Source: three-view drawing plus pictorial views. Frame: mm from the lowest corner of the part. A direction names the side the tool comes from. Give positions to 0.01 mm unless a question says otherwise; leave off trailing zeros. Order: outer loops, then holes, each group sorted by start corner. A loop starts at its lowest first (then second) coordinate and runs counter-clockwise, first axis right, second up. Notation, with made-up numbers: M 47.5,60.5 L 97.5,60.5 A19 ccw 97.5,84.5 Z; hole C -37,83 d9. An arc over 180 degrees is marked long. Use CSV: the item, a comma, the result in double quotes. Start each with the question number.
Item 1: First-contact query: pin 1 (4.5 mm diameter, centred on x = 11.575, y = 8.875, fed in from +Z); pin 2 (0.5 mm diameter, centred on x = 16, y = 9, fed in from +Z); pin 3 (2 mm diameter, centred on y = 17, z = 3, fed in from -X). Flat tips, straight axial feed; report the tip coordinate or a pass-through.
Item 2: Access query for the marked faces 1 and 2. Directions: +Z, -Z, +X, -X, +Y, -Y. A direction counts if a zero-diameter tool reaches every point of the face in a straight line with its end or side. Return the directions, or none.
Item 3: Ray query, probe 1 along X at (y, z) = (18.5, 2.9); probe 2 along Y at (x, z) = (13.25, 1.6); probe 3 along X at (y, z) = (9.25, 3.95). Return the intervals inside material, ascending. Write a range as from..to.
Item 4: Section query B-B on x = 12.5. Return loops of the section in (y, z).
Item 5: Section query C-C on y = 10.75. Return loops of the section in (x, z).
Item 6: Pull-direction query (X, two-part tool) for the marked faces 3, 4, 5 and 6; classes: +X half, -X half, draft (parallel to the pull), parting line (faces both ways), or undercut.
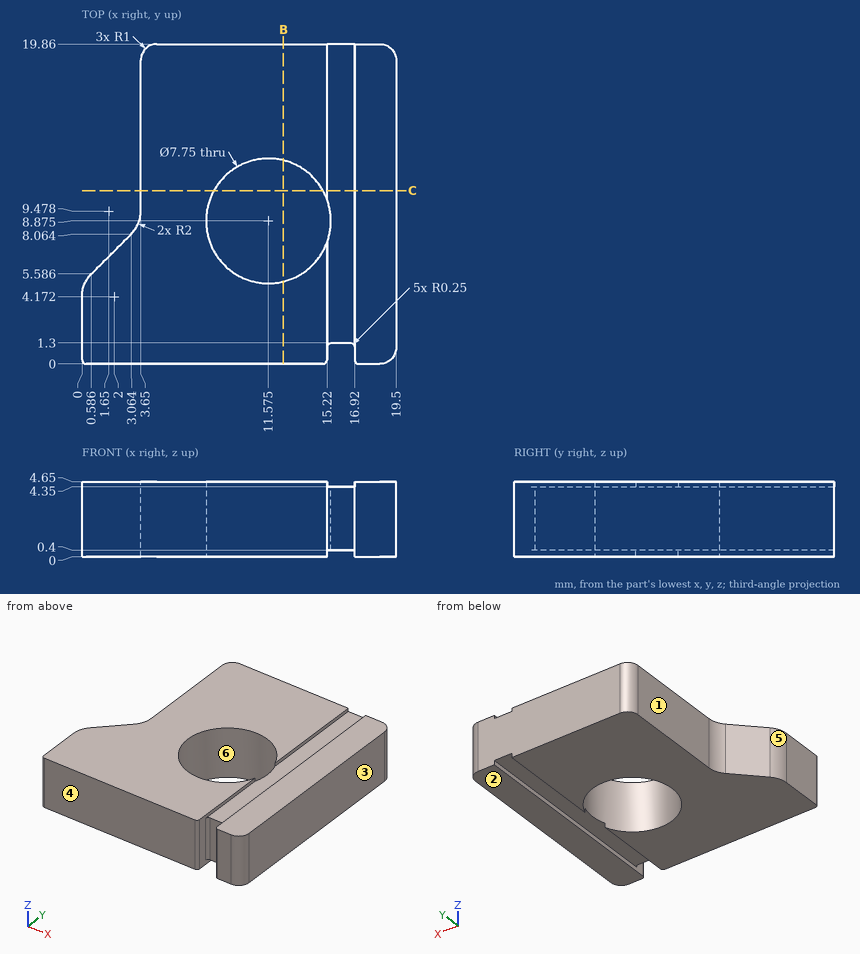
Verdict:
1,pin 1,"through"
1,pin 2,"z = 4.35"
1,pin 3,"x = 3.65"
2,face 1,"+Z, -Z, -X, +Y"
2,face 2,"-Z, +X, -X, +Y, -Y"
3,probe 1,"3.65..19.5"
3,probe 2,"0..5.38, 12.37..19.86"
3,probe 3,"3.64..7.72, 15.43..19.5"
4,outline,"M 0,0 L 5.11,0 L 5.11,4.65 L 0,4.65 Z; M 12.64,0 L 19.86,0 L 19.86,4.65 L 12.64,4.65 Z"
5,outline,"M 3.65,0 L 8.18,0 L 8.18,4.65 L 3.65,4.65 Z; M 14.97,0 L 15.22,0 L 15.22,0.4 L 16.92,0.4 L 16.92,0 L 19.5,0 L 19.5,4.65 L 16.92,4.65 L 16.92,4.35 L 15.22,4.35 L 15.22,4.65 L 14.97,4.65 Z"
6,face 3,"+X half"
6,face 4,"draft"
6,face 5,"-X half"
6,face 6,"undercut"
